Model file for the job. Use its own axes, mm. A direction names the side the tool comes from. Coordinates: 2 decimals unless noted, no trailing zeros. Loops run counter-clockwise (first coordinate to the right, second up) from the corner with the lowest first, then second, coordinate; pieces in that order, holes last.
Autodesk Fusion 360 part; units mm, degrees
sketch "Base" plane through (0, 0, 0) normal (0, 0, 1) x (1, 0, 0) in component " Thermistor Silicon Mold"
  line L0 (0, 0) -> (42, 0)
  line L1 (42, 0) -> (42, 12)
  line L2 (42, 12) -> (0, 12)
  line L3 (0, 12) -> (0, 0)
  dimension "d1" = 42
  dimension "d2" = 12
extrude "Extrude1" add sketch "Base" along normal blind 5.6 in component " Thermistor Silicon Mold"
fillet "Fillet1" radius 3 4 edges at (0, 0, 2.8) (42, 0, 2.8) (42, 12, 2.8) (0, 12, 2.8) in component " Thermistor Silicon Mold"
sketch "Hollow" plane through (0, 0, 5.6) normal (0, 0, 1) x (-1, 0, 0) in component " Thermistor Silicon Mold"
  arc A0 (-3, -12) -> (0, -9) centre (-3, -9) ccw
  line L0 (0, -9) -> (0, -3)
  arc A1 (0, -3) -> (-3, 0) centre (-3, -3) ccw
  line L1 (-3, 0) -> (-39, 0)
  arc A2 (-39, 0) -> (-42, -3) centre (-39, -3) ccw
  line L2 (-42, -3) -> (-42, -9)
  arc A3 (-42, -9) -> (-39, -12) centre (-39, -9) ccw
  line L3 (-39, -12) -> (-3, -12)
  line L4 (-1, -9) -> (-1, -3)
  arc A4 (-1, -3) -> (-3, -1) centre (-3, -3) ccw
  line L5 (-3, -1) -> (-39, -1)
  arc A5 (-39, -1) -> (-41, -3) centre (-39, -3) ccw
  line L6 (-41, -3) -> (-41, -9)
  arc A6 (-41, -9) -> (-39, -11) centre (-39, -9) ccw
  line L7 (-39, -11) -> (-3, -11)
  arc A7 (-3, -11) -> (-1, -9) centre (-3, -9) ccw
  dimension "d7" = -1
extrude "Extrude2" cut sketch "Hollow" against normal up to surface (5.6 mm away) contours L4 A4 L5 A5 L6 A6 L7 A7 in component " Thermistor Silicon Mold"
sketch "Hole" plane through (0, 0, 0) normal (-1, 0, 0) x (0, -1, 0) in component " Thermistor Silicon Mold"
  line L0 (-9, 5.6) -> (-9, 0)
  line L1 (-9, 0) -> (-3, 0)
  line L2 (-3, 0) -> (-3, 5.6)
  line L3 (-3, 5.6) -> (-9, 5.6)
  line L4 (-6, 5.6) -> (-6, 0) construction
  line L5 (-9, 2.8) -> (-3, 2.8) construction
  circle A0 centre (-6, 2.8) radius 1.5
  dimension "d10" = 3
extrude "Extrude3" cut sketch "Hole" against normal up to surface (1 mm away) contours A0 in component " Thermistor Silicon Mold"
sketch "Cut Through" plane through (0, 0, 0) normal (-1, 0, 0) x (0, -1, 0) in component " Thermistor Silicon Mold"
  circle A0 centre (-6, 2.8) radius 1.5
  line L0 (-9, 5.6) -> (-9, 0)
  line L1 (-9, 0) -> (-3, 0)
  line L2 (-3, 0) -> (-3, 5.6)
  line L3 (-3, 5.6) -> (-9, 5.6)
  line L4 (-6, 5.6) -> (-6, 0) construction
  line L5 (-6, 5.6) -> (-6.2, 5.6)
  line L6 (-6, 5.6) -> (-5.8, 5.6)
  line L7 (-6.2, 5.6) -> (-6.2, 0)
  line L8 (-5.8, 5.6) -> (-5.8, 0)
  line L9 (-6.2, 0) -> (-5.8, 0)
  dimension "d13" = 0.2
  dimension "d14" = 0.2
extrude "Extrude4" cut sketch "Cut Through" against normal up to surface (1 mm away) contours A0 L3 L5 L6 L7 L8 | A0 L1 L7 L8 L9 in component " Thermistor Silicon Mold"
component " Thermistor Silicon Mold" placed x (1, 0, 0) y (0, 1, 0) z (0, 0, 1) at (-1.1446, -0.9044, -0.1917)
Q1. Slice it at A-A (x = 6). List the corners of the cut face in (y, z).
Answers:
outline: (-0.9, -0.19) - (0.1, -0.19) - (0.1, 5.41) - (-0.9, 5.41) - close; (10.1, -0.19) - (11.1, -0.19) - (11.1, 5.41) - (10.1, 5.41) - close
Q2. Drill centre lines: line 1 (X direction, y = 8, z = 3.2); line 2 (Y direction, x = 12.5, z = 2.25); line 3 (X direction, y = 9, z = 2.9). Where is each one in solid material? Low to high.
Answers:
line 1: x = -1.14 to -0.14, 39.86 to 40.86
line 2: y = -0.9 to 0.1, 10.1 to 11.1
line 3: x = -1.01 to 0.07, 39.64 to 40.72
Q3. Slice it at B-B (y = 1). List the corners of the cut face in (x, z), and give its area (3 significant figures).
Answers:
outline: (-0.94, -0.19) - (0.18, -0.19) - (0.18, 5.41) - (-0.94, 5.41) - close; (39.53, -0.19) - (40.65, -0.19) - (40.65, 5.41) - (39.53, 5.41) - close
area: 12.5 mm2
Q4. Slice it at C-C (y = 6). List the corners of the cut face in (x, z), and give its area (3 significant figures).
Answers:
outline: (-1.14, -0.19) - (-0.14, -0.19) - (-0.14, 1.41) - (-1.14, 1.41) - close; (-1.14, 3.8) - (-0.14, 3.8) - (-0.14, 5.41) - (-1.14, 5.41) - close; (39.86, -0.19) - (40.86, -0.19) - (40.86, 5.41) - (39.86, 5.41) - close
area: 8.81 mm2
Q5. Flat gauge pins, fed straight in: P1, Ø0.8, axis at x = -0.5, z = 0.5, coming from the +Y side; P2, Ø1.1, axis at x = -0.5, z = 4.5, coming from the +Y side; P3, Ø1.1, axis at x = -1, z = 4.5, coming from the -Y side. Where does each tip first touch, or does it go through?
Answers:
P1: stops at y = 10.37
P2: stops at y = 10.49
P3: stops at y = 0.18
Q6. Slice it at D-D (z = 1.75). List the corners of the cut face in (x, y), and give its area (3 significant figures).
Answers:
outline: (-1.14, 2.1) arc R3 ccw to (1.86, -0.9) - (37.86, -0.9) arc R3 ccw to (40.86, 2.1) - (40.86, 8.1) arc R3 ccw to (37.86, 11.1) - (1.86, 11.1) arc R3 ccw to (-1.14, 8.1) - (-1.14, 6.33) - (-0.14, 6.33) - (-0.14, 8.1) arc R2 cw to (1.86, 10.1) - (37.86, 10.1) arc R2 cw to (39.86, 8.1) - (39.86, 2.1) arc R2 cw to (37.86, 0.1) - (1.86, 0.1) arc R2 cw to (-0.14, 2.1) - (-0.14, 3.87) - (-1.14, 3.87) - close
area: 97.2 mm2
Q7. Mould opens along Z. For faces 5 (the flat face through (-1.145, 3, 3)), 6 (the cylindrical face through (-0.652, 3.596, 2.578)) say: +Z half, -Z half, draft (parallel to the pull), parting line (faces both ways), or undercut.
Answers:
face 5: draft
face 6: undercut
Q8. Which spindle directions (+Z, -Z, +X, -X, +Y, -Y) get a long thin tool onto all of the face, cutting with end or side? Do faces 1 (the cylindrical face through (-0.652, 6.595, 2.638)), 2 (the cylindrical face through (39.29, 9.49, 2.65)), 3 (the cylindrical face through (-0.29, 0, 2.65)), 4 (the flat face through (-0.7, 5.296, 0.5)). Say none if no direction does.
Answers:
face 1: -X
face 2: +Z, -Z
face 3: +Z, -Z, -X, -Y
face 4: +Z, -Z, -X
